Verification items for the finished model (mm, model axes). A direction names the side the tool comes from. Coordinates: 2 decimals unless noted, no trailing zeros. Order: outer loops, then holes, each group sorted by start corner. A loop starts at its lowest first (then second) coordinate and runs counter-clockwise, first axis right, second up. Notation, with made-up numbers: (-20.5, 68) -> (17.5, 68) arc R16 cw to (17.5, 73) -> close; hole circle Ø10 at (-10, 13). An arc over 180 degrees is marked (long way). Use CSV: the item, a comma, the result in double quotes. Start each with the question number.
1) Sectioned sample at A-A on y = 11. Record the boundary of the cut face in (x, z), then the cut area to 3 significant figures.
2) Sectioned sample at C-C on x = 16. Record the boundary of the cut face in (y, z), then the cut area to 3 significant figures.
3) Sectioned sample at D-D on x = 2. Record the boundary of the cut face in (y, z).
4) Release check for a two-part mould opening along X. For faces 1 (the cylindrical face through (-32, 6, 0)), 2 (the cylindrical face through (-11.46, 1.52, 2.3)), 3 (the flat face through (20, 33, 3)) record: released by +X, released by -X, zero draft, split by the parting line, or undercut.
5) Scan lines: line 1 along X through (y, z) = (2.35, 0); line 2 along Z through (x, y) = (-17, 3.6); line 3 along Z through (x, y) = (17, 26.5). Record each from-to range of solid material in increasing order.
6) Sectioned sample at B-B on z = 0. Record the boundary of the cut face in (x, y).
7) Tool access check on faces 4 (the cylindrical face through (32, 6, 0)), 5 (the flat face through (13, 9, -8)). Record the directions out of +Z, -Z, +X, -X, +Y, -Y that give a thin tool (end or side, any length) a straight path to the whole face; none if there is none.
8) Go/stop test with flat-tipped pins: pin 1 (2 mm diameter, centred on y = 8.5, z = 9, fed in from -X); pin 2 (10 mm diameter, centred on x = -3.5, z = -7, fed in from +Y); pin 3 (8 mm diameter, centred on y = 19, z = -5, fed in from +X). Record where each tip stops, or that it passes through.
from build123d import *

# Parameters (mm, degrees)
BOSS_EXTRUDE1_DEPTH = 12
CUT_EXTRUDE1_DEPTH  = 7
SKETCH3_R           = 6
SKETCH3_R_2         = 3.5
BOSS_EXTRUDE2_DEPTH = 28
SKETCH4_R           = 3.5
CUT_EXTRUDE2_DEPTH  = 28
SKETCH5_R           = 8
SKETCH5_R_2         = 6
CUT_EXTRUDE3_DEPTH  = 2
SKETCH5_3_R         = 6
CUT_EXTRUDE4_DEPTH  = 6


with BuildPart() as part:
    # Sketch1 → Boss-Extrude1 (new body)
    with BuildSketch(Plane(origin=(0, 0, 0), x_dir=(1, 0, 0), z_dir=(0, 1, 0))):
        with BuildLine():
            Line((-17, 15), (17, 15))
            ThreePointArc((17, 15), (32, 0), (17, -15))
            Line((17, -15), (-17, -15))
            ThreePointArc((-17, -15), (-32, 0), (-17, 15))
        make_face()
    extrude(amount=BOSS_EXTRUDE1_DEPTH)

    # Sketch2 → Cut-Extrude1 (cut)
    with BuildSketch(Plane(origin=(0, 12, 0), x_dir=(1, 0, 0), z_dir=(0, 1, 0))):
        with BuildLine():
            Line((8, 10), (-17, 10))
            ThreePointArc((-17, 10), (-27, 0), (-17, -10))
            Line((-17, -10), (8, -10))
            Line((8, -10), (8, -8))
            Line((8, -8), (17, -8))
            ThreePointArc((17, -8), (25, 0), (17, 8))
            Line((17, 8), (8, 8))
            Line((8, 8), (8, 10))
        make_face()
    extrude(amount=-CUT_EXTRUDE1_DEPTH, mode=Mode.SUBTRACT)

    # Sketch3 → Boss-Extrude2 (add)
    with BuildSketch(Plane(origin=(0, 5, 0), x_dir=(1, 0, 0), z_dir=(0, 1, 0))):
        with Locations((17, 0)):
            Circle(SKETCH3_R)
        with Locations((17, 0)):
            Circle(SKETCH3_R_2, mode=Mode.SUBTRACT)
    extrude(amount=BOSS_EXTRUDE2_DEPTH)

    # Sketch4 → Cut-Extrude2 (cut)
    with BuildSketch(Plane(origin=(0, 5, 0), x_dir=(1, 0, 0), z_dir=(0, 1, 0))):
        with Locations((17, 0)):
            Circle(SKETCH4_R)
    extrude(amount=-CUT_EXTRUDE2_DEPTH, mode=Mode.SUBTRACT)

    # Sketch5 → Cut-Extrude3 (cut)
    with BuildSketch(Plane(origin=(0, 5, 0), x_dir=(1, 0, 0), z_dir=(0, 1, 0))):
        with Locations((-17, 0)):
            Circle(SKETCH5_R)
        with Locations((-17, 0)):
            Circle(SKETCH5_R_2, mode=Mode.SUBTRACT)
    extrude(amount=-CUT_EXTRUDE3_DEPTH, mode=Mode.SUBTRACT)

    # Sketch5_3 → Cut-Extrude4 (cut, through all)
    with BuildSketch(Plane(origin=(0, 5, 0), x_dir=(1, 0, 0), z_dir=(0, 1, 0))):
        with Locations((-17, 0)):
            Circle(SKETCH5_3_R)
    extrude(amount=-CUT_EXTRUDE4_DEPTH, mode=Mode.SUBTRACT)


solid = part.part
Answers follow:
1,outline,"(-17, -15) -> (17, -15) arc R15 ccw to (17, 15) -> (-17, 15) arc R15 ccw to start; circle Ø12 at (17, 0); hole (-17, -10) -> (8, -10) -> (8, -8) -> (17, -8) arc R8 ccw to (17, 8) -> (8, 8) -> (8, 10) -> (-17, 10) arc R10 ccw to start; hole circle Ø7 at (17, 0)"
1,area,"900 mm²"
2,outline,"(0, -15) -> (12, -15) -> (12, -8) -> (5, -8) -> (5, -5.92) -> (33, -5.92) -> (33, -3.35) -> (0, -3.35) -> close; (0, 3.35) -> (33, 3.35) -> (33, 5.92) -> (5, 5.92) -> (5, 8) -> (12, 8) -> (12, 15) -> (0, 15) -> close"
2,area,"358 mm²"
3,outline,"(0, -15) -> (12, -15) -> (12, -10) -> (5, -10) -> (5, 10) -> (12, 10) -> (12, 15) -> (0, 15) -> close"
4,face 1,"released by -X"
4,face 2,"undercut"
4,face 3,"zero draft"
5,line 1,"x = -32 to -23, -11 to 13.5, 20.5 to 32"
5,line 2,"z = -15 to -8, 8 to 15"
5,line 3,"z = -6 to -3.5, 3.5 to 6"
6,outline,"(-32, 0) -> (-23, 0) -> (-23, 3) -> (-25, 3) -> (-25, 5) -> (-27, 5) -> (-27, 12) -> (-32, 12) -> close; (-11, 0) -> (13.5, 0) -> (13.5, 33) -> (11, 33) -> (11, 5) -> (-9, 5) -> (-9, 3) -> (-11, 3) -> close; (20.5, 0) -> (32, 0) -> (32, 12) -> (25, 12) -> (25, 5) -> (23, 5) -> (23, 33) -> (20.5, 33) -> close"
7,face 4,"+X, +Y, -Y"
7,face 5,"+Y"
8,pin 1,"stops at x = -29.69"
8,pin 2,"stops at y = 12"
8,pin 3,"stops at x = 22.92"
